Autodesk Inventor part; units mm, degrees
ref_plane "YZ Plane" through (0, 0, 0) normal (1, 0, 0) x (0, 1, 0)
ref_plane "XZ Plane" through (0, 0, 0) normal (0, 1, 0) x (-1, 0, 0)
ref_plane "XY Plane" through (0, 0, 0) normal (0, 0, 1) x (1, 0, 0)
sketch "Sketch1" plane through (0, 0, 0) normal (0, 1, 0) x (-1, 0, 0)
  line L0 (-12.065, 21.59) -> (12.065, 21.59)
  line L1 (12.065, 21.59) -> (12.065, -21.59)
  line L2 (12.065, -21.59) -> (-12.065, -21.59)
  line L3 (-12.065, -21.59) -> (-12.065, 21.59)
  line L4 (-12.065, 21.59) -> (12.065, -21.59) construction
  line L5 (12.065, 21.59) -> (-12.065, -21.59) construction
  line L6 (-9.652, 19.177) -> (9.652, 19.177)
  line L7 (9.652, 19.177) -> (9.652, -19.177)
  line L8 (9.652, -19.177) -> (-9.652, -19.177)
  line L9 (-9.652, -19.177) -> (-9.652, 19.177)
  line L10 (-9.652, 19.177) -> (9.652, -19.177) construction
  line L11 (9.652, 19.177) -> (-9.652, -19.177) construction
  point P0 (0, 0)
  dimension "d0" = 24.13
  dimension "d1" = 43.18
  dimension "d2" = 19.304
  dimension "d3" = 38.354
extrude "Extrusion1" add sketch "Sketch1" along normal blind 3.81
extrude "Extrusion2" add sketch "Sketch1" against normal blind 2.54 contours L0 L1 L2 L3 | L6 L7 L8 L9
sketch "Sketch2" plane through (-9.652, 3.81, 19.177) normal (1, 0, 0) x (0, 0, -1)
  line L0 (19.177, -3.81) -> (19.177, -1.016)
  dimension "d8" = 2.794
hole "Hole1" at (-9.652, 2.794, 0) direction (-1, 0, 0) diameter 3.302 end through all both
fillet "Fillet1" radius 3.175 4 edges at (0, -2.54, -21.59) (12.065, -2.54, 0) (-12.065, -2.54, 0) (0, -2.54, 21.59)
properties part number "HomemadeSensorHousing 8020-Lid"
Can you work these out from the model? Positions are in its coordinate system, mm. A direction names the side the tool comes from. Round coordinates to 2 decimals unless told otherwise and drop trailing zeros. Write each loop counter-clockwise with the first axis right and the second up, starting at its lowest first coordinate (ties: lowest second). Pieces come first, ordered by that corner, then holes. Notation, with made-up numbers: (50.5, -37.75) -> (72.5, -37.75) arc R22 cw to (72.5, -21.75) -> close; hole circle Ø7 at (17.25, 11). An arc over 180 degrees is marked (long way). Use one line per item in the form item = value. Start each with the question number.
Q1. Imagine slicing it at C-C (x = 1). Please give me the cut outline in (y, z) (3 decimals).
Q2. Imagine slicing it at D-D (y = -1.25). Please give me the cut outline in (x, z).
Q3. We'd pull the mould along Z, two halves only. Please class faces 3 (the face through (0, 2, -21.59)), 4 (the face through (1, 3.81, 20)), 5 (the face through (-9.652, 1, 0.3)): +Z half, -Z half, draft (parallel to the pull), parting line (faces both ways), or undercut.
Q4. Which directions (+Z, -Z, +X, -X, +Y, -Y) give clear straight access to the entire face, cutting with the end or side of a thin tool? Please do faces 1 (the face through (0, 2, 19.177)), 2 (the face through (11.11, -1.635, 0.302)).
Q5. Imagine slicing it at A-A (y = 1.75). Please give me the cut outline in (x, z) (3 decimals).
Q6. I'm going to push flat-ended pins straight in: P1, Ø2, axis at y = -1.5, z = -10, coming from the +X side; P2, Ø6, axis at x = -2, z = -2.5, coming from the +Y side; P3, Ø1.5, axis at x = -7.5, y = 0, coming from the -Z side. Where does each tip first touch, or does it pass through?
Q7. Imagine slicing it at B-B (z = -3). Please give me the cut outline in (x, y) (3 decimals), then the cut area to 3 significant figures.
Q8. If I drill on probe 1 along X at (y, z) = (3, -18) (3 decimals); probe 2 along Z at (x, y) = (-3.5, 1.5); probe 3 along Y at (x, z) = (5.5, 13.5), over which ranges is the centre line in solid material (lowest first)? Write a range as [from, to].
Worked out:
q1.outline = (-2.54, -18.415) arc R3.175 ccw to (0.635, -21.59) -> (3.81, -21.59) -> (3.81, -19.177) -> (0, -19.177) -> (0, 19.177) -> (3.81, 19.177) -> (3.81, 21.59) -> (0.635, 21.59) arc R3.175 ccw to (-2.54, 18.415) -> close
q2.outline = (-11.44, -20.97) -> (11.44, -20.97) -> (11.44, 20.97) -> (-11.44, 20.97) -> close
q3.face_3 = -Z half
q3.face_4 = draft
q3.face_5 = undercut
q4.face_1 = +Y
q4.face_2 = +Z, -Z, +X, -Y
q5.outline = (-12.065, -21.59) -> (12.065, -21.59) -> (12.065, -1.279) -> (9.652, -1.279) -> (9.652, -19.177) -> (-9.652, -19.177) -> (-9.652, -1.279) -> (-12.065, -1.279) -> close; (-12.065, 1.279) -> (-9.652, 1.279) -> (-9.652, 19.177) -> (9.652, 19.177) -> (9.652, 1.279) -> (12.065, 1.279) -> (12.065, 21.59) -> (-12.065, 21.59) -> close
q6.P1 = 11.86
q6.P2 = 0
q6.P3 = -21.59
q7.outline = (-12.065, 0.635) arc R3.175 ccw to (-8.89, -2.54) -> (8.89, -2.54) arc R3.175 ccw to (12.065, 0.635) -> (12.065, 3.81) -> (9.652, 3.81) -> (9.652, 0) -> (-9.652, 0) -> (-9.652, 3.81) -> (-12.065, 3.81) -> close
q7.area = 75.4 mm^2
q8.probe_1 = [-12.065, -9.652], [9.652, 12.065]
q8.probe_2 = [-21.59, -19.18], [19.18, 21.59]
q8.probe_3 = [-2.54, 0]
